```python
from build123d import *

# Parameters (mm, degrees)
SKETCH1_W                       = 7
SKETCH1_H                       = 7
SKETCH1_R                       = 2
BOSS_EXTRUDE1_DEPTH             = 20
BOSS_EXTRUDE2_REACH             = 5.5
SKETCH2_W                       = 7
SKETCH2_H                       = 6
SKETCH2_R                       = 1.5
BOSS_EXTRUDE2_DIRECTION_2_REACH = 5.5


with BuildPart() as part:
    # Sketch1 → Boss-Extrude1 (new body)
    with BuildSketch(Plane(origin=(0, 0, 0), x_dir=(1, 0, 0), z_dir=(0, 1, 0))):
        Rectangle(SKETCH1_W, SKETCH1_H)
        Circle(SKETCH1_R, mode=Mode.SUBTRACT)
    extrude(amount=BOSS_EXTRUDE1_DEPTH)

    # Boss-Extrude2: up to this face of the body (flat: up to its plane)
    boss_extrude2_end = Plane(part.part.faces().sort_by_distance((0, 10, 3.5))[0])
    # Sketch2 → Boss-Extrude2 (add, up to the picked face)
    with BuildSketch(Plane.XY, mode=Mode.PRIVATE) as boss_extrude2_sk1:
        with Locations((0, 23)):
            Rectangle(SKETCH2_W, SKETCH2_H)
        with Locations((0, 23)):
            Circle(SKETCH2_R, mode=Mode.SUBTRACT)
    boss_extrude2_tool1 = split(extrude(boss_extrude2_sk1.sketch, amount=BOSS_EXTRUDE2_REACH, mode=Mode.PRIVATE), bisect_by=boss_extrude2_end, keep=Keep.BOTH, mode=Mode.PRIVATE)
    add(boss_extrude2_tool1.solids().sort_by_distance((0, 25.907805, 0))[0])

    # Boss-Extrude2 direction 2: up to this face of the body (flat: up to its plane)
    boss_extrude2_direction_2_end = Plane(part.part.faces().sort_by_distance((0, 10, -3.5))[0])
    # Sketch2 → Boss-Extrude2 direction 2 (add, up to the picked face)
    with BuildSketch(Plane.XY, mode=Mode.PRIVATE) as boss_extrude2_direction_2_sk1:
        with Locations((0, 23)):
            Rectangle(SKETCH2_W, SKETCH2_H)
        with Locations((0, 23)):
            Circle(SKETCH2_R, mode=Mode.SUBTRACT)
    boss_extrude2_direction_2_tool1 = split(extrude(boss_extrude2_direction_2_sk1.sketch, amount=-BOSS_EXTRUDE2_DIRECTION_2_REACH, mode=Mode.PRIVATE), bisect_by=boss_extrude2_direction_2_end, keep=Keep.BOTH, mode=Mode.PRIVATE)
    add(boss_extrude2_direction_2_tool1.solids().sort_by_distance((0, 25.907805, 0))[0])


solid = part.part
```
Geometry: final body of the model. Coordinates: model frame, mm. A direction names the side the tool comes from. Round coordinates to 2 decimals unless told otherwise and drop trailing zeros. Write each loop counter-clockwise with the first axis right and the second up, starting at its lowest first coordinate (ties: lowest second). Pieces come first, ordered by that corner, then holes. Notation, with made-up numbers: M 21,63 L 48,63 A35 ccw 48,97 Z; hole C 81.25,-15.75 d2. An arc over 180 degrees is marked long. Answer in a Markdown table with one row per item. Add a question column.
(1) Cut plane A-A, the plane y = 23. Return the cut outline in (x, z), then the cut area to 3 significant figures.
(2) Reachability of faces 4 (the face through (-0.195, 24.487, 0.049)), 5 (the face through (0, 10, 2)) from +Z, -Z, +X, -X, +Y, -Y: full face, straight path, thin tool, end or side. Return the list, or none.
(3) Cut plane B-B, the plane x = 0. Return the cut outline in (y, z), then the cut area to 3 significant figures.
(4) Draft query along X for faces 1 (the face through (0, 13, 3.5)), 2 (the face through (0, 20, 0)), 3 (the face through (-3.5, 13, 0)). Return one class per face: pulls with the +X half, pulls with the -X half, needs draft (parallel to the pull), parting line crosses it, or undercut.
(5) Cut plane C-C, the plane y = 16.5. Return the cut outline in (x, z).
(6) Ray query, L1, parallel to X at y = 5.5, z = 0; L2, parallel to Y at x = 0, z = -1. Return the intervals inside material, ascending.
(7) Cut plane D-D, the plane z = 1.5. Return the cut outline in (x, y), then the cut area to 3 significant figures.
Established:
| question | item | result |
|---|---|---|
| 1 | outline | M -3.5,-3.5 L -1.5,-3.5 L -1.5,3.5 L -3.5,3.5 Z; M 1.5,-3.5 L 3.5,-3.5 L 3.5,3.5 L 1.5,3.5 Z |
| 1 | area | 28.0 mm² |
| 2 | face 4 | +Z, -Z |
| 2 | face 5 | -Y |
| 3 | outline | M 0,-3.5 L 21.5,-3.5 L 21.5,3.5 L 0,3.5 L 0,2 L 20,2 L 20,-2 L 0,-2 Z; M 24.5,-3.5 L 26,-3.5 L 26,3.5 L 24.5,3.5 Z |
| 3 | area | 81.0 mm² |
| 4 | face 1 | needs draft |
| 4 | face 2 | undercut |
| 4 | face 3 | pulls with the -X half |
| 5 | outline | M -3.5,-3.5 L 3.5,-3.5 L 3.5,3.5 L -3.5,3.5 Z; hole C 0,0 d4 |
| 6 | L1 | -3.5 to -2, 2 to 3.5 |
| 6 | L2 | 20 to 21.5, 24.5 to 26 |
| 7 | outline | M -3.5,0 L -1.32,0 L -1.32,20 L 1.32,20 L 1.32,0 L 3.5,0 L 3.5,26 L -3.5,26 Z; hole C 0,23 d3 |
| 7 | area | 122 mm² |
